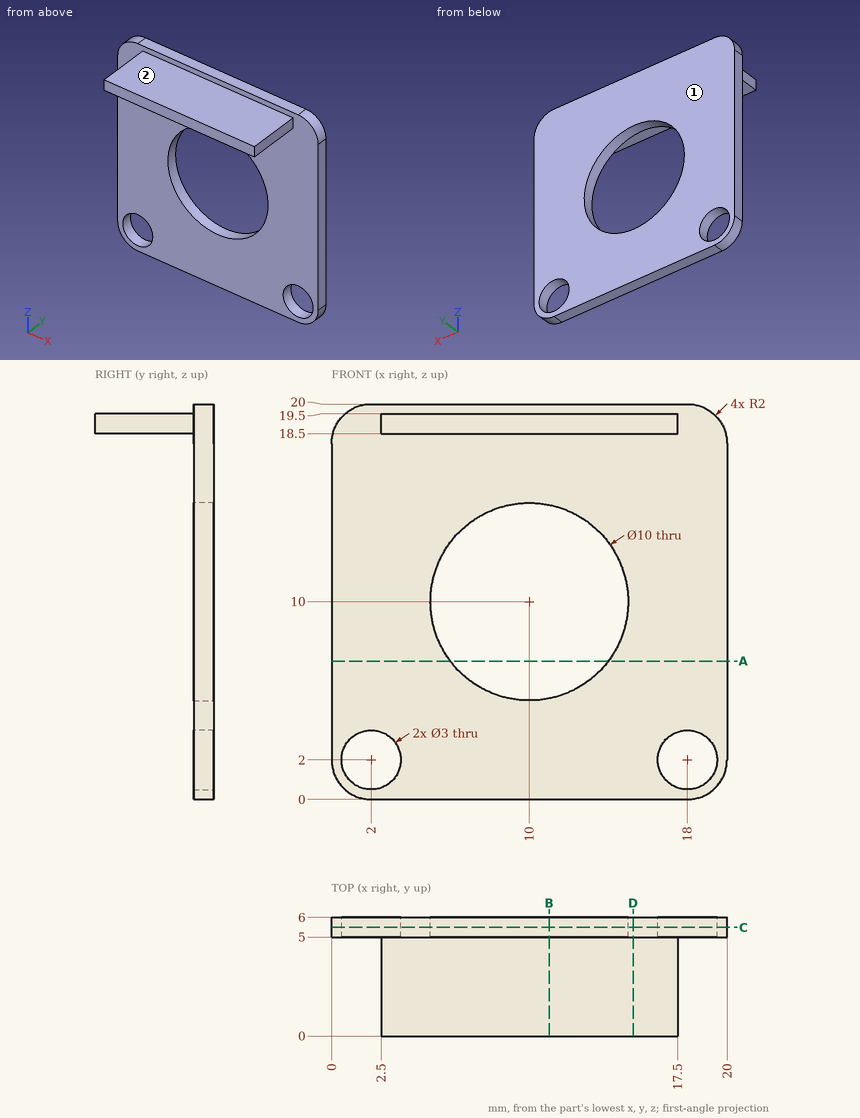
Geometry check sheet. Reference: drawing and pictorial views, mm from the part's lowest x, y, z. A direction names the side the tool comes from. Round coordinates to 2 decimals unless told otherwise and drop trailing zeros. Loops run counter-clockwise (first coordinate to the right, second up) from the corner with the lowest first, then second, coordinate; pieces in that order, holes last. Notation, with made-up numbers: (17.25, 74.25) -> (76.25, 74.25) arc R25 ccw to (76.25, 98.25) -> close; hole circle Ø4 at (-35.5, 36.25). An arc over 180 degrees is marked (long way). Answer as a JSON object with one key per item and string values. Group by question number.
Item 1: Depth check by flat-ended pin: pin 1 Ø1.5 at (x, y) = (17.5, 4) entering from -Z; pin 2 Ø4 at (x, z) = (2, 2) entering from -Y; pin 3 Ø1.1 at (y, z) = (1.5, 19) entering from +X. Enter the tip coordinate at first touch or a pass-through.
Item 2: Set-up check for the marked faces 1 and 2: record each of +Z, -Z, +X, -X, +Y, -Y from which the full face is reachable in a straight line by a thin tool's end or side.
Item 3: Cross-section at D-D, the plane x = 15.25. Record the cut outline in (y, z).
Item 4: Cross-section at B-B, the plane x = 11. Record the cut outline in (y, z), plus the area to 3 significant figures.
Item 5: Cross-section at C-C, the plane y = 5.5. Record the cut outline in (x, z), plus the area to 3 significant figures.
Item 6: Thickness scan on line 1 along X through (y, z) = (5.4, 2); line 2 along X through (y, z) = (5.3, 10); line 3 along Y through (x, z) = (6, 5.25). Record the ranges inside material, lowest first.
Item 7: Cross-section at A-A, the plane z = 7. Record the cut outline in (x, y), plus the area to 3 significant figures.
Determined:
{
 "1": {"pin 1": "stops at z = 18.5", "pin 2": "stops at y = 5", "pin 3": "stops at x = 17.5"},
 "2": {"face 1": "+Z, -Z, +X, -X, +Y", "face 2": "+Z, +X, -X, -Y"},
 "3": {"outline": "(0, 18.5) -> (5, 18.5) -> (5, 0) -> (6, 0) -> (6, 20) -> (5, 20) -> (5, 19.5) -> (0, 19.5) -> close"},
 "4": {"outline": "(0, 18.5) -> (5, 18.5) -> (5, 14.9) -> (6, 14.9) -> (6, 20) -> (5, 20) -> (5, 19.5) -> (0, 19.5) -> close; (5, 0) -> (6, 0) -> (6, 5.1) -> (5, 5.1) -> close", "area": "15.2 mm²"},
 "5": {"outline": "(0, 2) arc R2 ccw to (2, 0) -> (18, 0) arc R2 ccw to (20, 2) -> (20, 18) arc R2 ccw to (18, 20) -> (2, 20) arc R2 ccw to (0, 18) -> close; hole circle Ø3 at (2, 2); hole circle Ø10 at (10, 10); hole circle Ø3 at (18, 2)", "area": "304 mm²"},
 "6": {"line 1": "x = 0 to 0.5, 3.5 to 16.5, 19.5 to 20", "line 2": "x = 0 to 5, 15 to 20", "line 3": "y = 5 to 6"},
 "7": {"outline": "(0, 5) -> (6, 5) -> (6, 6) -> (0, 6) -> close; (14, 5) -> (20, 5) -> (20, 6) -> (14, 6) -> close", "area": "12.0 mm²"}
}
